Verification items for the finished model (mm, model axes). A direction names the side the tool comes from. Round coordinates to 2 decimals unless told otherwise and drop trailing zeros. Order: outer loops, then holes, each group sorted by start corner. A loop starts at its lowest first (then second) coordinate and runs counter-clockwise, first axis right, second up. Notation, with made-up numbers: M 16.5,80.5 L 58.5,80.5 A26 cw 58.5,116.5 Z; hole C 34.25,47.25 d3. An arc over 180 degrees is marked long. Use CSV: the item, a comma, the result in double quotes. Start each with the question number.
Q1. Gauge pin test, flat ends, axial feed: pin 1 Ø1.5 at (x, z) = (19.5, 2) entering from +Y; pin 2 Ø0.9 at (x, z) = (8, 1) entering from -Y. Record the tip position at first contact, or that the pin passes through.
Q2. Scan lines: line 1 (Y direction, x = -1, z = 1.15); line 2 (Y direction, x = -24.5, z = 1.7); line 3 (X direction, y = 13.5, z = 0.65). Record each from-to range of solid material in increasing order.
Q3. Mould release check, pull along X, two halves, no side actions. Record for faces 5 (the face through (-40, 1, 1)), 6 (the face through (-37, 79.5, 1)), 7 (the face through (4.04, 0, 1)): +X half, -X half, draft (parallel to the pull), parting line (faces both ways), or undercut.
Q4. Sectioned sample at A-A (x = 12). Enter the section's corners in (y, z), and give its area (3 significant figures).
Q5. Set-up check for faces 1 (the face through (-10, -78, 1)), 2 (the face through (0, 79.5, 1)), 3 (the face through (-13, -1.5, 1)), 4 (the face through (-22, 78, 1)): record each of +Z, -Z, +X, -X, +Y, -Y from which the full face is reachable in a straight line by a thin tool's end or side.
Q6. Sectioned sample at D-D (z = 2.55). State how many separate pieces and enclosed holes the cut face has, and give its area (3 significant figures).
Q7. Sectioned sample at C-C (x = 0). Enter the section's corners in (y, z).
Q8. Sectioned sample at B-B (y = -11). Enter the section's corners in (x, z).
```python
from build123d import *

# Parameters (mm, degrees)
SKETCH1_W           = 6
SKETCH1_H           = 3
SKETCH1_W_2         = 3
SKETCH1_H_2         = 6
BOSS_EXTRUDE1_DEPTH = 3


with BuildPart() as part:
    # Sketch1 → Boss-Extrude1 (new body)
    with BuildSketch(Plane.XY):
        Polygon((-34, 76.5), (-28, 76.5), (-28, 79.5), (-22, 79.5), (-22, 76.5), (-16, 76.5), (-16, 79.5), (-10, 79.5), (-10, 76.5), (-4, 76.5), (-4, 79.5), (0, 79.5), (4, 79.5), (4, 76.5), (10, 76.5), (10, 79.5), (16, 79.5), (16, 76.5), (22, 76.5), (22, 79.5), (28, 79.5), (28, 76.5), (34, 76.5), (34, 79.5), (40, 79.5), (40, 76.5), (40, -76.5), (40, -79.5), (34, -79.5), (34, -76.5), (28, -76.5), (28, -79.5), (22, -79.5), (22, -76.5), (16, -76.5), (16, -79.5), (10, -79.5), (10, -76.5), (4, -76.5), (4, -79.5), (0, -79.5), (-4, -79.5), (-4, -76.5), (-10, -76.5), (-10, -79.5), (-16, -79.5), (-16, -76.5), (-22, -76.5), (-22, -79.5), (-28, -79.5), (-28, -76.5), (-34, -76.5), (-34, -79.5), (-40, -79.5), (-40, -76.5), (-40, 76.5), (-40, 79.5), (-34, 79.5), align=None)
        Polygon((-1.503424482, 2.54), (1.503424482, 2.54), (1.503424482, 1.5), (4.04, 1.5), (4.04, -1.5), (1.503424482, -1.5), (1.503424482, -2.54), (-1.503424482, -2.54), (-1.503424482, -1.5), (-4.04, -1.5), (-4.04, 1.5), (-1.503424482, 1.5), align=None, mode=Mode.SUBTRACT)
        with Locations((25.04, 0)):
            Rectangle(SKETCH1_W, SKETCH1_H, mode=Mode.SUBTRACT)
        with Locations((-13.04, 0)):
            Rectangle(SKETCH1_W, SKETCH1_H, mode=Mode.SUBTRACT)
        with Locations((-25.04, 0)):
            Rectangle(SKETCH1_W, SKETCH1_H, mode=Mode.SUBTRACT)
        with Locations((13.04, 0)):
            Rectangle(SKETCH1_W, SKETCH1_H, mode=Mode.SUBTRACT)
        with Locations((0, -23.54)):
            Rectangle(SKETCH1_W_2, SKETCH1_H_2, mode=Mode.SUBTRACT)
        with Locations((0, 11.54)):
            Rectangle(SKETCH1_W_2, SKETCH1_H_2, mode=Mode.SUBTRACT)
        with Locations((0, 23.54)):
            Rectangle(SKETCH1_W_2, SKETCH1_H_2, mode=Mode.SUBTRACT)
        with Locations((0, -11.54)):
            Rectangle(SKETCH1_W_2, SKETCH1_H_2, mode=Mode.SUBTRACT)
    extrude(amount=BOSS_EXTRUDE1_DEPTH)


solid = part.part
```
Verdict:
1,pin 1,"stops at y = 76.5"
1,pin 2,"stops at y = -76.5"
2,line 1,"y = -79.5 to -26.54, -20.54 to -14.54, -8.54 to -2.54, 2.54 to 8.54, 14.54 to 20.54, 26.54 to 79.5"
2,line 2,"y = -79.5 to -1.5, 1.5 to 79.5"
2,line 3,"x = -40 to -1.5, 1.5 to 40"
3,face 5,"-X half"
3,face 6,"draft"
3,face 7,"undercut"
4,outline,"M -79.5,0 L -1.5,0 L -1.5,3 L -79.5,3 Z; M 1.5,0 L 79.5,0 L 79.5,3 L 1.5,3 Z"
4,area,"468 mm²"
5,face 1,"+Z, -Z, -Y"
5,face 2,"+Z, -Z, +X, -X, +Y"
5,face 3,"+Z, -Z"
5,face 4,"+Z, -Z, +Y"
6,separate pieces,"1"
6,enclosed holes,"9"
6,area,"12,300 mm²"
7,outline,"M -79.5,0 L -26.54,0 L -26.54,3 L -79.5,3 Z; M -20.54,0 L -14.54,0 L -14.54,3 L -20.54,3 Z; M -8.54,0 L -2.54,0 L -2.54,3 L -8.54,3 Z; M 2.54,0 L 8.54,0 L 8.54,3 L 2.54,3 Z; M 14.54,0 L 20.54,0 L 20.54,3 L 14.54,3 Z; M 26.54,0 L 79.5,0 L 79.5,3 L 26.54,3 Z"
8,outline,"M -40,0 L -1.5,0 L -1.5,3 L -40,3 Z; M 1.5,0 L 40,0 L 40,3 L 1.5,3 Z"
